from build123d import *

# Parameters (mm, degrees)
F0_W        = 9.3987649307
F0_H        = 84.1068960726
F1_DEPTH    = 3.048
F2_T1_DEPTH = 107.386380603
F3_DEPTH    = 16.764


# Not quite as in the source:
# - a fillet or chamfer that OpenCascade refuses, or shapes differently, is made with other operations: its cross-section is extruded or revolved along the edge and cut away or added


with BuildPart() as f1:
    # F0 (on Front) → F1 (new body)
    with BuildSketch(Plane.XZ):
        with Locations((-10.7242320664, -3.0124243349)):
            Rectangle(F0_W, F0_H)
    extrude(amount=F1_DEPTH)

    # F2: fillet of radius 5.08 on 2 edges, made by hand

    # F2_s2 → F2_t1 (cut)
    with BuildSketch(Plane.XY.offset(-56.7056146364)):
        with BuildLine():
            ThreePointArc((-6.0248496011, -3.048), (-7.898315915, -0.8297670652), (-10.6807465072, 0))
            Line((-10.6807465072, 0), (-6.0248496011, 0))
            Line((-6.0248496011, 0), (-6.0248496011, -3.048))
        make_face()
        with BuildLine():
            ThreePointArc((-15.4236145318, -3.048), (-13.5501482178, -0.8297670652), (-10.7677176257, 0))
            Line((-10.7677176257, 0), (-15.4236145318, 0))
            Line((-15.4236145318, 0), (-15.4236145318, -3.048))
        make_face()
    extrude(amount=F2_T1_DEPTH, mode=Mode.SUBTRACT)

    # F3 (add): a face of the model
    f3_faces = [f1.faces().sort_by_distance(p)[0] for p in [
        (-10.7242320664, -1.7873359361, 39.0410237014),
    ]]
    extrude(f3_faces, amount=F3_DEPTH)


solid = f1.part
Can you work these out from the model? Positions are in its coordinate system, mm. Give positions to 0.01 mm unless a question says otherwise; leave off trailing zeros. Write each loop counter-clockwise with the first axis right and the second up, starting at its lowest first coordinate (ties: lowest second). Pieces come first, ordered by that corner, then holes. Notation, with made-up numbers: (26.5, 28.5) -> (81.5, 28.5) arc R19 cw to (81.5, 56.5) -> close; hole circle Ø10 at (62.25, -17). An arc over 180 degrees is marked (long way). Answer as a JSON object with one key per item and string values. Group by question number.
Item 1: Suppose I cut it at A-A (z = 36.5). Please give me the cut outline in (x, y).
Item 2: Suppose I cut it at B-B (y = -0.7). Please give me the cut outline in (x, z), plus the area to 3 significant figures.
Item 3: Please list where these lines run through material, in increasing order: line 1 (Y direction, x = -10.25, z = 14); line 2 (Y direction, x = -12.75, z = -7.5); line 3 (X direction, y = -1.8, z = -28). Write a range as [from, to].
Findings:
{
 "1": {"outline": "(-15.42, -3.05) -> (-6.02, -3.05) arc R5.08 ccw to (-10.68, 0) -> (-10.77, 0) arc R5.08 ccw to start"},
 "2": {"outline": "(-13.34, -45.07) -> (-8.11, -45.07) -> (-8.11, 55.81) -> (-13.34, 55.81) -> close", "area": "528 mm²"},
 "3": {"line 1": "y = [-3.05, -0.02]", "line 2": "y = [-3.05, -0.4]", "line 3": "x = [-14.65, -6.8]"}
}
